Autodesk Inventor part; units mm, degrees
ref_plane "Work Plane1" through (-10.4775, -10.4775, 12.7) normal (0, 0, 1) x (1, 0, 0)
ref_plane "YZ Plane" through (0, 0, 0) normal (1, 0, 0) x (0, 1, 0)
ref_plane "XZ Plane" through (0, 0, 0) normal (0, 1, 0) x (-1, 0, 0)
sketch "Sketch1" plane through (0, 0, 0) normal (0, 0, 1) x (1, 0, 0)
  circle A0 centre (0, 0) radius 4.191
  circle A1 centre (0, 0) radius 4.191
  point P0 (0, 0)
ref_plane "Work Plane1" through (-10.4775, -10.4775, 12.7) normal (0, 0, 1) x (1, 0, 0)
extrude "Extrusion1" add sketch "Sketch1" along normal blind 17.145
sketch "Sketch2" plane through (0, 0, 17.145) normal (0, 0, 1) x (1, 0, 0)
  circle A0 centre (0, 0) radius 4.191
  line L0 (-2.0955, -3.6295) -> (-4.191, 0)
  line L1 (-4.191, 0) -> (-2.0955, 3.6295)
  line L2 (-2.0955, 3.6295) -> (2.0955, 3.6295)
  line L3 (2.0955, 3.6295) -> (4.191, 0)
  line L4 (4.191, 0) -> (2.0955, -3.6295)
  line L5 (2.0955, -3.6295) -> (-2.0955, -3.6295)
  point P0 (0, 0)
  point P1 (0, 0)
extrude "Extrusion2" add sketch "Sketch2" along normal blind 13.97 contours L4 L5 L0 L1 L2 L3
sketch "Sketch3" plane through (0, 0, 31.115) normal (0, 0, 1) x (1, 0, 0)
  circle A0 centre (0, 0) radius 1.905
  dimension "d4" = 3.81
extrude "Extrusion3" add sketch "Sketch3" along normal blind 8.89
properties part number "Wheel_Pin"
Here's how the part is built. I have some questions about the finished solid (model axes, mm). A direction names the side the tool comes from. Coordinates: 2 decimals unless noted, no trailing zeros. Order: outer loops, then holes, each group sorted by start corner. A loop starts at its lowest first (then second) coordinate and runs counter-clockwise, first axis right, second up. Notation, with made-up numbers: M -35.5,13 L -1.5,13 A28 ccw -1.5,38 Z; hole C 46,-16.75 d3. An arc over 180 degrees is marked long. Answer as CSV lines item,"result".
Item 1: On a 3-axis mill with a long thin cutter (end or side, diameter ignored), from which of +Z, -Z, +X, -X, +Y, -Y can I reach the whole of each face in a straight line? I mean faces 1 (the face through (0, -3.63, 24)), 2 (the face through (-3.158, 1.789, 24.032)), 3 (the face through (3.158, -1.789, 24.032)), 4 (the face through (-3.4, -1.8, 17.145)), 5 (the face through (3.13, 1.84, 24.03)). Say none if no direction works.
Results found:
face 1,"+Z, +X, -X, -Y"
face 2,"+Z, -X, +Y"
face 3,"+Z, +X, -Y"
face 4,"+Z, -X, -Y"
face 5,"+Z, +X, +Y"
Item 2: Imagine slicing it at A-A on x = 0. Write out the boundary of the cut face in (y, z) (1 decimal).
Results found:
outline,"M -4.2,0 L 4.2,0 L 4.2,17.1 L 3.6,17.1 L 3.6,31.1 L 1.9,31.1 L 1.9,40 L -1.9,40 L -1.9,31.1 L -3.6,31.1 L -3.6,17.1 L -4.2,17.1 Z"
Item 3: Imagine slicing it at D-D on z = 13. Write out the boundary of the cut face in (x, y).
Results found:
outline,"C 0,0 d8.38"
Item 4: Imagine slicing it at B-B on z = 29. Write out the boundary of the cut face in (x, y).
Results found:
outline,"M -4.19,0 L -2.1,-3.63 L 2.1,-3.63 L 4.19,0 L 2.1,3.63 L -2.1,3.63 Z"
Item 5: For pin 1 (1.7 mm diameter, centred on x = -3.5, y = -1.5, fed in from +Z) (3 decimals); pin 2 (4 mm diameter, centred on x = -2, z = 20, fed in from -Y); pin 3 (3 mm diameter, centred on x = -0.5, y = 2, fed in from -Z); pin 4 (0.6 mm diameter, centred on x = 0, y = 4, fed in from +Z) (3 decimals), each with a flat end and sliding along its axis, tell me the tip position at first contact or that it passes through.
Results found:
pin 1,"z = 31.115"
pin 2,"y = -3.63"
pin 3,"z = 0"
pin 4,"z = 17.145"
Item 6: If I drill on line 1 (Y direction, x = -0.25, z = 8); line 2 (Z direction, x = -2, y = 2) (3 decimals); line 3 (Z direction, x = 3.75, y = 1) (3 decimals), over which ranges is the centre line in solid material (lowest first)?
Results found:
line 1,"-4.18 to 4.18"
line 2,"0 to 31.115"
line 3,"0 to 17.145"
Item 7: Imagine slicing it at C-C on y = -3. Write out the boundary of the cut face in (x, z) (3 decimals).
Results found:
outline,"M -2.927,0 L 2.927,0 L 2.927,17.145 L 2.459,17.145 L 2.459,31.115 L -2.459,31.115 L -2.459,17.145 L -2.927,17.145 Z"
